For this review, take the finished solid that the model builds, in its own axes (mm). A direction names the side the tool comes from. Coordinates: 2 decimals unless noted, no trailing zeros. Write each loop counter-clockwise with the first axis right and the second up, starting at its lowest first coordinate (ties: lowest second). Pieces come first, ordered by that corner, then holes.
1) Insertion check: P1, Ø5, axis at x = -2.5, z = 16, coming from the +Y side; P2, Ø1, axis at y = -2.5, z = 14, coming from the +X side; P3, Ø6, axis at x = 4, z = 22, coming from the +Y side. Each pin has a flat end and moves straight along its axis. Give the tip position at first contact, or say it passes through.
2) To check wall thickness, follow line 1 along Y through (x, z) = (0, 6) (3 decimals); line 2 along Z through (x, y) = (-5.25, 1). State the ranges of each line that lie inside material, in increasing order.
3) We need section A-A on x = 0. Write out the cut boundary in (y, z) (3 decimals).
4) For faces 5 (the face through (0, 4, 2)), 6 (the face through (-4, 0.25, 4)), 7 (the face through (-4, -0.25, 4)), 8 (the face through (-0.6, 2.6, 17)), list the 3-axis set-ups (+Z, -Z, +X, -X, +Y, -Y) from which the entire face can be reached by the end or side of a thin tool; tool diameter is ignored.
5) We need section C-C on x = 4.25. Write out the cut boundary in (y, z), then the cut area to 3 significant figures.
6) We need section B-B on z = 17.75. Write out the cut boundary in (x, y) (3 decimals).
7) Mouldability with a two-part tool opening along X and no side actions: class faces 1 (the face through (1.5, -2.8, 13.3)), 2 (the face through (0, -4, 2)), 3 (the face through (-0.6, -2.6, 17)), 4 (the face through (4.563, -0.003, 4.994)) as pulls with the +X half, pulls with the -X half, needs draft (parallel to the pull), parting line crosses it, or undercut.
8) We need section D-D on y = -3.5. Write out the cut boundary in (x, z).
from build123d import *

# Parameters (mm, degrees)
SKETCH001_R     = 6
PAD_DEPTH       = 2
SKETCH_R        = 3.175
SKETCH_R_2      = 2.25
PAD001_DEPTH    = 25
PAD002_DEPTH    = 0.25
SKETCH005_W     = 1.2
SKETCH005_H     = 6.35
POCKET_DEPTH    = 21.176
SKETCH006_R     = 2.25
POCKET001_DEPTH = 28.118792


with BuildPart() as part:
    # Sketch001 → Pad (new body)
    with BuildSketch(Plane.XY):
        Circle(SKETCH001_R)
    extrude(amount=PAD_DEPTH)

    # Sketch → Pad001 (join)
    with BuildSketch(Plane.XY):
        Circle(SKETCH_R)
        Circle(SKETCH_R_2, mode=Mode.SUBTRACT)
    extrude(amount=PAD001_DEPTH)

    # Sketch002 → Pad002 (join, symmetric)
    with BuildSketch(Plane.XZ):
        Polygon((-6, 2), (0, 14.5), (6, 2), align=None)
    extrude(amount=PAD002_DEPTH, both=True)

    # Sketch004 → Revolution (revolve)
    with BuildSketch(Plane.XZ):
        with BuildLine():
            ThreePointArc((3.175, 25), (2.245064, 27.245064), (0, 28.175))
            Line((0, 25), (0, 28.175))
            Line((0, 25), (3.175, 25))
        make_face()
    revolve(axis=Axis((0, 0, 0), (0, 0, 1)))

    # Sketch005 → Pocket (cut, through all)
    with BuildSketch(Plane.XY.offset(7)):
        Rectangle(SKETCH005_W, SKETCH005_H)
    extrude(amount=POCKET_DEPTH, mode=Mode.SUBTRACT)

    # Sketch006 → Pocket001 (cut, through all)
    with BuildSketch(Plane.XY):
        Circle(SKETCH006_R)
    extrude(amount=POCKET001_DEPTH, mode=Mode.SUBTRACT)


solid = part.part
Result:
1. P1: stops at y = 3.12
1. P2: stops at x = 2.47
1. P3: stops at y = 3.01
2. line 1: y = -3.175 to -2.25, 2.25 to 3.175
2. line 2: z = 0 to 2
3. outline: (-6, 0) - (-2.25, 0) - (-2.25, 7) - (-3.175, 7) - (-3.175, 2) - (-6, 2) - close; (2.25, 0) - (6, 0) - (6, 2) - (3.175, 2) - (3.175, 7) - (2.25, 7) - close
4. face 5: +Z, +Y
4. face 6: +Z, -X, +Y
4. face 7: +Z, -X, -Y
4. face 8: +Z, +Y, -Y
5. outline: (-4.24, 0) - (4.24, 0) - (4.24, 2) - (0.25, 2) - (0.25, 5.65) - (-0.25, 5.65) - (-0.25, 2) - (-4.24, 2) - close
5. area: 18.8 mm2
6. outline: (-0.6, -3.118) - (-0.6, -2.169) arc R2.25 cw to (-0.6, 2.169) - (-0.6, 3.118) arc R3.175 ccw to start; (0.6, -3.118) arc R3.175 ccw to (0.6, 3.118) - (0.6, 2.169) arc R2.25 cw to (0.6, -2.169) - close
7. face 1: parting line crosses it
7. face 2: needs draft
7. face 3: undercut
7. face 4: pulls with the +X half
8. outline: (-4.87, 0) - (4.87, 0) - (4.87, 2) - (-4.87, 2) - close
